Check sheet for the modelled part. Datum: model origin and axes. Units: mm. Coordinates: 2 decimals unless noted, no trailing zeros. Write each loop counter-clockwise with the first axis right and the second up, starting at its lowest first coordinate (ties: lowest second). Pieces come first, ordered by that corner, then holes. Notation, with made-up numbers: (72.5, 12) -> (111.5, 12) arc R5 cw to (111.5, 18) -> close; hole circle Ø9 at (85, 72.5). An arc over 180 degrees is marked (long way). One line per item, written item: value. Start each with the question number.
1) Sectioned sample at C-C on z = -1.15. Enter the section's corners in (x, y).
2) Scan lines: line 1 along X through (y, z) = (-1, -0.65); line 2 along X through (y, z) = (-0.9, 0.6); line 3 along Z through (x, y) = (-2.75, 0.3). Record each from-to range of solid material in increasing order. Write a range as [from, to].
3) Sectioned sample at A-A on z = 0. Enter the section's corners in (x, y).
4) Sectioned sample at D-D on x = 0.75. Enter the section's corners in (y, z).
5) Gauge pin test, flat end, axial feed: P1, Ø1, axis at x = -2.5, z = -0.5, coming from the -Y side. Record the tip position at first contact, or that the pin passes through.
```python
from build123d import *

# Parameters (mm, degrees)
F0_R     = 1
F1_DEPTH = 2
F3_ANGLE = 180


# Not quite as in the source:
# - a pattern or mirror of a feature is missing from the dataset's text; its kind, count and spacing are read off the source's solid


with BuildPart() as f1:
    # F0 (on Right) → F1 (new body, symmetric)
    with BuildSketch(Plane.YZ):
        Circle(F0_R)
    extrude(amount=F1_DEPTH, both=True)

    # F2 (on face) → F3 (revolve)
    with BuildSketch(Plane.YZ.offset(2)):
        with BuildLine():
            Line((0, -1.5), (0, 1.5))
            ThreePointArc((0, 1.5), (-1.5, 0), (0, -1.5))
        make_face()
    f3 = revolve(axis=Axis((2, 0, 0), (0, 0, 1)), revolution_arc=F3_ANGLE)

    # F3_copies: F3 across plane
    add(f3.mirror(Plane(origin=(0, 0, 0), x_dir=(0, 0, -1), z_dir=(-1, 0, 0))))


solid = f1.part
```
Answers:
1. outline: (-2, -0.96) -> (-2, 0.96) arc R0.96 ccw to start; (2, -0.96) arc R0.96 ccw to (2, 0.96) -> close
2. line 1: x = [-2.91, -2], [2, 2.91]
2. line 2: x = [-3.04, -2], [2, 3.04]
2. line 3: z = [-1.26, 1.26]
3. outline: (-2, -1.5) -> (-2, -1) -> (2, -1) -> (2, -1.5) arc R1.5 ccw to (2, 1.5) -> (2, 1) -> (-2, 1) -> (-2, 1.5) arc R1.5 ccw to start
4. outline: circle Ø2 at (0, 0)
5. P1: stops at y = -1.49
